CAD build for the part. Positions are in the model's coordinates, mm. A direction names the side the tool comes from. Give positions to 0.01 mm unless a question says otherwise; leave off trailing zeros. Loops run counter-clockwise (first coordinate to the right, second up) from the corner with the lowest first, then second, coordinate; pieces in that order, holes last.
Item 1: Saw through at B-B on x = 19. Give the cut face in (y, z).
Item 2: Which spindle directions (+Z, -Z, +X, -X, +Y, -Y) get a long thin tool onto all of the face, cutting with end or side? Do faces 4 (the flat face through (5.796, 16.23, 7.507)), 5 (the flat face through (-16.95, -3.1, 0.49)), 6 (the flat face through (13.386, 1, 4)). Say none if no direction does.
Item 3: Saw through at C-C on z = 2. Give the number of separate pieces and of enclosed holes in the cut face, plus the area to 3 significant figures.
Item 4: Probe probe 1 along X at (y, z) = (-17.5, 4.75); probe 2 along X at (y, z) = (-6, 3.25); probe 3 along Y at (x, z) = (9.5, 4). List the from-to ranges inside material, lowest first.
Item 5: Mould opens along X. For faces 1 (the flat face through (-13.386, 2, 4)), 2 (the flat face through (-26.97, -21.54, 0.49)), 3 (the flat face through (11, 25, 4)) say: released by +X, released by -X, zero draft, split by the parting line, or undercut.
Item 6: Saw through at A-A on y = 27. Give the cut face in (x, z), plus the area to 3 significant figures.
Item 7: Drop flat-ended pins along their axis: P1, Ø1.5, axis at y = 10, z = 7, coming from the +X side; P2, Ø3, axis at y = 28, z = 5, coming from the -X side; P3, Ø1.8, axis at y = 0, z = 3.5, coming from the +X side. Give the stop position or say it passes through.
from build123d import *

# Parameters (mm, degrees)
F1_DEPTH = 8
F2_SIZE  = 1


# Not quite as in the source:
# - a feature names something its author has since deleted; it is built from what else it names


with BuildPart() as f1:
    # F0 (on Top) → F1 (new body)
    with BuildSketch(Plane.XY):
        Polygon((2.7355143452, 13.8776440214), (0, 12.2982940778), (-2.7355143452, 13.8776440214), (-13.3861494398, 7.7284969825), (-13.3861494398, -4.5697970953), (-10.6506350946, -6.1491470389), (-10.6506350946, -9.3078469261), (0, -15.456993965), (10.6506350946, -9.3078469261), (10.6506350946, -6.1491470389), (13.3861494398, -4.5697970953), (13.3861494398, 7.7284969825), align=None)
        with BuildLine():
            ThreePointArc((0, 11.25), (7.9549512883, 7.9549512883), (11.25, 0))
            ThreePointArc((11.25, 0), (-7.9549512883, -7.9549512883), (0, 11.25))
        make_face(mode=Mode.SUBTRACT)
        Polygon((-2.7355143452, 13.8776440214), (0, 12.2982940778), (0, 14.8963702892), (-0.4855143452, 15.1766821271), align=None)
        Polygon((0, 14.8963702892), (0, 12.2982940778), (2.7355143452, 13.8776440214), (0.4855143452, 15.1766821271), align=None)
        Polygon((-11, 18.6491470389), (-2.7355143452, 13.8776440214), (-0.4855143452, 15.1766821271), (-8.75, 19.9481851446), (-8.75, 30.0518148554), (0, 35.1036297108), (8.75, 30.0518148554), (8.75, 19.9481851446), (0.4855143452, 15.1766821271), (2.7355143452, 13.8776440214), (11, 18.6491470389), (11, 31.3508529611), (0, 37.7017059222), (-11, 31.3508529611), align=None)
        Polygon((-13.3861494398, -7.1678733067), (-13.3861494398, -4.5697970953), (-21.6506350946, 0.2017059222), (-32.6506350946, -6.1491470389), (-32.6506350946, -18.8508529611), (-21.6506350946, -25.2017059222), (-10.6506350946, -18.8508529611), (-10.6506350946, -9.3078469261), (-12.9006350946, -8.0088088204), (-12.9006350946, -17.5518148554), (-21.6506350946, -22.6036297108), (-30.4006350946, -17.5518148554), (-30.4006350946, -7.4481851446), (-21.6506350946, -2.3963702892), align=None)
        Polygon((-10.6506350946, -6.1491470389), (-13.3861494398, -4.5697970953), (-13.3861494398, -7.1678733067), (-12.9006350946, -7.4481851446), (-12.9006350946, -8.0088088204), (-10.6506350946, -9.3078469261), align=None)
        Polygon((13.3861494398, -7.1678733067), (13.3861494398, -4.5697970953), (10.6506350946, -6.1491470389), (10.6506350946, -9.3078469261), (12.9006350946, -8.0088088204), (12.9006350946, -7.4481851446), align=None)
        Polygon((21.6506350946, 0.2017059222), (13.3861494398, -4.5697970953), (13.3861494398, -7.1678733067), (21.6506350946, -2.3963702892), (30.4006350946, -7.4481851446), (30.4006350946, -17.5518148554), (21.6506350946, -22.6036297108), (12.9006350946, -17.5518148554), (12.9006350946, -8.0088088204), (10.6506350946, -9.3078469261), (10.6506350946, -18.8508529611), (21.6506350946, -25.2017059222), (32.6506350946, -18.8508529611), (32.6506350946, -6.1491470389), align=None)
    extrude(amount=F1_DEPTH)

    # F2
    f2_edges = [f1.edges().sort_by_distance(p)[0] for p in [
        (-8.060832, 10.803071, 8),
        (-13.386149, 1.57935, 8),
        (-17.518392, -2.184046, 8),
        (-27.150635, -2.973721, 8),
        (-32.650635, -12.5, 8),
        (-27.150635, -22.026279, 8),
        (-16.150635, -22.026279, 8),
        (-5.325318, -12.38242, 8),
        (-10.650635, -14.07935, 8),
        (5.325318, -12.38242, 8),
        (10.650635, -14.07935, 8),
        (16.150635, -22.026279, 8),
        (27.150635, -22.026279, 8),
        (32.650635, -12.5, 8),
        (27.150635, -2.973721, 8),
        (17.518392, -2.184046, 8),
        (13.386149, 1.57935, 8),
        (8.060832, 10.803071, 8),
        (6.867757, 16.263396, 8),
        (11, 25, 8),
        (5.5, 34.526279, 8),
        (-5.5, 34.526279, 8),
        (-11, 25, 8),
        (-6.867757, 16.263396, 8),
        (-11, 25, 0),
        (-5.5, 34.526279, 0),
        (5.5, 34.526279, 0),
        (11, 25, 0),
        (6.867757, 16.263396, 0),
        (-6.867757, 16.263396, 0),
        (-8.060832, 10.803071, 0),
        (8.060832, 10.803071, 0),
        (13.386149, 1.57935, 0),
        (-13.386149, 1.57935, 0),
        (17.518392, -2.184046, 0),
        (27.150635, -2.973721, 0),
        (32.650635, -12.5, 0),
        (27.150635, -22.026279, 0),
        (16.150635, -22.026279, 0),
        (10.650635, -14.07935, 0),
        (5.325318, -12.38242, 0),
        (-5.325318, -12.38242, 0),
        (-10.650635, -14.07935, 0),
        (-16.150635, -22.026279, 0),
        (-27.150635, -22.026279, 0),
        (-32.650635, -12.5, 0),
        (-27.150635, -2.973721, 0),
        (-17.518392, -2.184046, 0),
    ]]
    chamfer(f2_edges, length=F2_SIZE)


solid = f1.part
Results below:
1. outline: (-23.67, 1) - (-22.52, 0) - (-21.07, 0) - (-21.07, 8) - (-22.52, 8) - (-23.67, 7) - close; (-3.93, 0) - (-2.48, 0) - (-1.33, 1) - (-1.33, 7) - (-2.48, 8) - (-3.93, 8) - close
2. face 4: +Z, +X
2. face 5: -Z, +Y
2. face 6: +Z, -Z, +Y
3. separate pieces: 1
3. enclosed holes: 4
3. area: 659 mm2
4. probe 1: x = -32.65 to -30.4, -12.9 to -10.65, 10.65 to 12.9, 30.4 to 32.65
4. probe 2: x = -32.39 to -27.89, -15.41 to -9.52, 9.52 to 15.41, 27.89 to 32.39
4. probe 3: y = -9.97 to -6.03, 6.03 to 9.97, 17.78 to 32.22
5. face 1: undercut
5. face 2: released by -X
5. face 3: released by +X
6. outline: (-11, 1) - (-10, 0) - (-8.75, 0) - (-8.75, 8) - (-10, 8) - (-11, 7) - close; (8.75, 0) - (10, 0) - (11, 1) - (11, 7) - (10, 8) - (8.75, 8) - close
6. area: 34.0 mm2
7. P1: stops at x = 10.75
7. P2: stops at x = -11
7. P3: stops at x = 23.56
